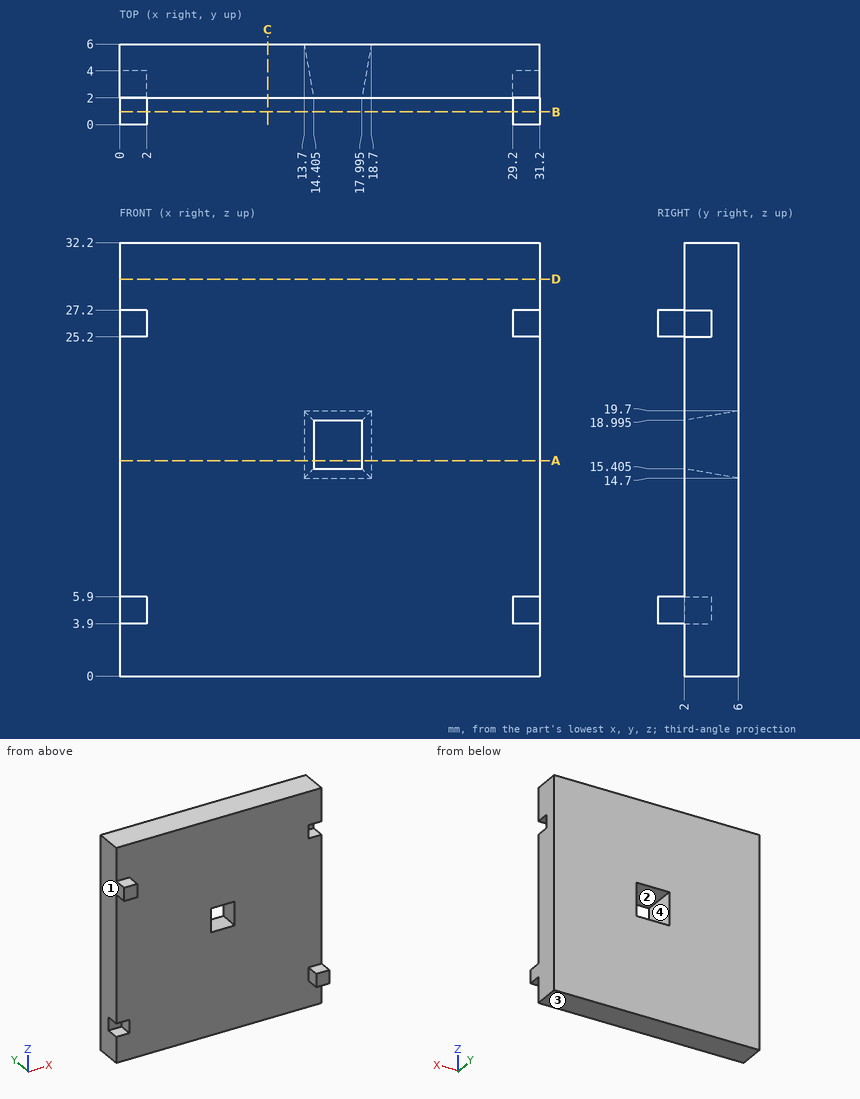
Verification items for this drawing (mm, ordinates from the low corner). Coordinates: 2 decimals unless noted, no trailing zeros. Loops run counter-clockwise (first coordinate to the right, second up) from the corner with the lowest first, then second, coordinate; pieces in that order, holes last. Notation, with made-up numbers: (-33, 33.5) -> (2, 33.5) arc R28 ccw to (2, 62.5) -> close; hole circle Ø2 at (-26, -37.75). An arc over 180 degrees is marked (long way). Answer in a Markdown table with one row per item. Add a question column.
1. Section check B-B, the plane y = 0.95. Enter the section's corners in (x, z).
2. Draft check along Z on the marked faces 1, 2, 3 and 4. Enter one of: +Z half, -Z half, draft (parallel to the pull), parting line (faces both ways), or undercut.
3. Section check A-A, the plane z = 16. Enter the section's corners in (x, y) (1 decimal), then the cut area to 3 significant figures.
4. Depth check by flat-ended pin: P1, Ø2, axis at x = 1, z = 5, coming from the -Y side; P2, Ø1.6, axis at x = 1, y = 3, coming from the -Z side; P3, Ø0.6, axis at x = 30, y = 1, coming from the -Z side; P4, Ø0.6, axis at x = 30.5, y = 1, coming from the +Z side. Enter the tip coordinate at first touch or a pass-through.
5. Section check C-C, the plane x = 11. Enter the section's corners in (y, z), then the cut area to 3 significant figures.
6. Section check D-D, the plane z = 29.5. Enter the section's corners in (x, y).
7. Material ranges on probe 1 along Y at (x, z) = (27, 30.5); probe 2 along X at (y, z) = (3.3, 4); probe 3 along X at (y, z) = (5.65, 15.5), recorded low to high. Write a range as [from, to].
Derived:
| question | item | result |
|---|---|---|
| 1 | outline | (0, 25.2) -> (2, 25.2) -> (2, 27.2) -> (0, 27.2) -> close; (29.2, 3.9) -> (31.2, 3.9) -> (31.2, 5.9) -> (29.2, 5.9) -> close |
| 2 | face 1 | draft |
| 2 | face 2 | undercut |
| 2 | face 3 | -Z half |
| 2 | face 4 | undercut |
| 3 | outline | (0, 2) -> (14.4, 2) -> (13.7, 6) -> (0, 6) -> close; (18, 2) -> (31.2, 2) -> (31.2, 6) -> (18.7, 6) -> close |
| 3 | area | 108 mm² |
| 4 | P1 | stops at y = 2 |
| 4 | P2 | stops at z = 0 |
| 4 | P3 | stops at z = 3.9 |
| 4 | P4 | stops at z = 5.9 |
| 5 | outline | (2, 0) -> (6, 0) -> (6, 32.2) -> (2, 32.2) -> close |
| 5 | area | 129 mm² |
| 6 | outline | (0, 2) -> (31.2, 2) -> (31.2, 6) -> (0, 6) -> close |
| 7 | probe 1 | y = [2, 6] |
| 7 | probe 2 | x = [2, 31.2] |
| 7 | probe 3 | x = [0, 13.76], [18.64, 31.2] |
